from build123d import *

# Parameters (mm, degrees)
F1_DEPTH      = 76.2
F3_DEPTH      = 25.4
F3_DEPTH_BACK = 25.4
F5_START      = -19.05
F4_R          = 15.875
F5_DEPTH      = 15.494
F7_DEPTH      = 25.908
F10_DEPTH     = 6.35


with BuildPart() as f1:
    # F0 (on Front) → F1 (new body, symmetric)
    with BuildSketch(Plane.XZ):
        Polygon((-76.2, 0), (0, 0), (0, 152.4), (-25.4, 152.4), (-25.4, 25.4), (-76.2, 25.4), align=None)
    extrude(amount=F1_DEPTH, both=True)

    # F2 (on Right) → F3 (cut, two sides)
    with BuildSketch(Plane.YZ) as f3_sk:
        with BuildLine():
            ThreePointArc((0, 114.3), (4.4901280605, 116.1598719395), (6.35, 120.65))
            ThreePointArc((6.35, 120.65), (-4.4901280605, 125.1401280605), (0, 114.3))
        make_face()
    extrude(amount=-F3_DEPTH, mode=Mode.SUBTRACT)
    extrude(f3_sk.sketch, amount=F3_DEPTH_BACK, mode=Mode.SUBTRACT)

    # F4 (on Right) → F5 (cut)
    with BuildSketch(Plane.YZ.offset(F5_START)):
        with Locations((0, 120.65)):
            Circle(F4_R)
    extrude(amount=-F5_DEPTH, mode=Mode.SUBTRACT)

    # F6 (on Top) → F7 (cut, symmetric)
    with BuildSketch(Plane.XY):
        with BuildLine():
            Line((-76.2, 12.7), (-76.2, 0))
            Line((-76.2, 0), (-76.2, -12.7))
            Line((-76.2, -12.7), (-63.5, -12.7))
            ThreePointArc((-63.5, -12.7), (-50.8, 0), (-63.5, 12.7))
            Line((-63.5, 12.7), (-76.2, 12.7))
        make_face()
    extrude(amount=F7_DEPTH, both=True, mode=Mode.SUBTRACT)

    # F9 (on offset) → F10 (join, symmetric)
    with BuildSketch(Plane.XZ.offset(44.45)):
        Polygon((-50.8, 25.4), (-25.4, 25.4), (-25.4, 101.6), align=None)
    extrude(amount=F10_DEPTH, both=True)


solid = f1.part
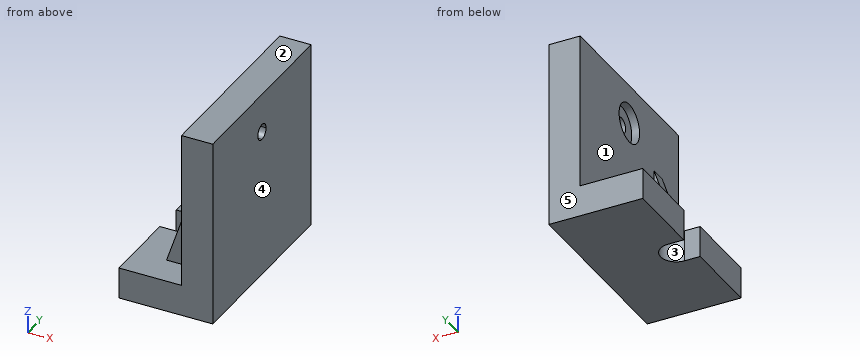
For this review, take the finished solid that the model builds, in its own axes (mm). Face numbers are marked on the shaded views. A direction names the side the tool comes from. Give positions to 0.01 mm unless a question says otherwise; leave off trailing zeros. Loops run counter-clockwise (first coordinate to the right, second up) from the corner with the lowest first, then second, coordinate; pieces in that order, holes last. Notation, with made-up numbers: M 87.5,82.25 L 93.5,82.25 A20 ccw 93.5,94.25 Z; hole C -11.5,49.25 d3. An arc over 180 degrees is marked long. Put each result on its own line as item: value. Start each with the question number.
(1) Add section B-B, the plane y = -2. Write out the cut boundary in (x, z).
(2) For pin 1 (10 mm diameter, centred on x = -30.5, y = 53, fed in from +Z); pin 2 (7.5 mm diameter, centred on x = -43.5, z = 57.5, fed in from -Y); pin 3 (16 mm diameter, centred on y = -5, z = 118, fed in from -X), all flat-tipped, find the tip position at first contact; note any pin that passes through.
(3) Wall thickness on L1, parallel to Y at x = -20, z = 120; L2, parallel to Z at x = -22, y = 0 (3 decimals); L3, parallel to Y at x = -10.75, z = 120.65: over which ranges is each line inside the solid? List them lowest first.
(4) Add section A-A, the plane x = -58. Write out the cut boundary in (y, z).
(5) Add section D-D, the plane x = -45. Write out the cut boundary in (y, z).
(6) Add section C-C, the plane z = 123. Write out the cut boundary in (x, y).
(7) The part is to be moulded in two halves that separate along Y. For the marked faces 3, 4 and 5, say which applies: +Y half, -Y half, draft (parallel to the pull), parting line (faces both ways), or undercut.
(8) Machinability: for the marked faces 1 and 2, which of the approach directions +Z, -Z, +X, -X, +Y, -Y give a long, thin tool a straight path to every point of the face, cutting with its end or side? Answer none if there is none.
Result:
1. outline: M -50.96,0 L 0,0 L 0,114.62 L -19.05,114.62 L -19.05,104.9 L -25.4,104.9 L -25.4,25.4 L -50.96,25.4 Z; M -25.4,136.4 L -19.05,136.4 L -19.05,126.68 L 0,126.68 L 0,152.4 L -25.4,152.4 Z
2. pin 1: stops at z = 25.4
2. pin 2: stops at y = -50.8
2. pin 3: stops at x = -19.05
3. L1: y = -76.2 to -15.86, 15.86 to 76.2
3. L2: z = 0 to 104.775, 136.525 to 152.4
3. L3: y = -76.2 to -6.35, 6.35 to 76.2
4. outline: M -76.2,0 L -11.45,0 L -11.45,25.4 L -76.2,25.4 Z; M 11.45,0 L 76.2,0 L 76.2,25.4 L 11.45,25.4 Z
5. outline: M -76.2,0 L 76.2,0 L 76.2,25.4 L -38.1,25.4 L -38.1,42.8 L -50.8,42.8 L -50.8,25.4 L -76.2,25.4 Z
6. outline: M -25.4,-76.2 L 0,-76.2 L 0,-5.9 L -19.05,-5.9 L -19.05,-15.7 L -25.4,-15.7 Z; M -25.4,15.7 L -19.05,15.7 L -19.05,5.9 L 0,5.9 L 0,76.2 L -25.4,76.2 Z
7. face 3: undercut
7. face 4: draft
7. face 5: +Y half
8. face 1: +Z, -X
8. face 2: +Z, +X, -X, +Y, -Y
